Autodesk Inventor part; units mm, degrees
ref_plane "YZ Plane" through (0, 0, 0) normal (1, 0, 0) x (0, 1, 0)
ref_plane "XZ Plane" through (0, 0, 0) normal (0, 1, 0) x (-1, 0, 0)
ref_plane "XY Plane" through (0, 0, 0) normal (0, 0, 1) x (1, 0, 0)
sketch "スケッチ1" plane through (0, 0, 0) normal (0, 1, 0) x (-1, 0, 0)
  line L0 (19, -14) -> (-19, -14)
  line L1 (-19, -14) -> (-19, 14)
  line L2 (-19, 14) -> (19, 14)
  line L3 (19, 14) -> (19, -14)
  line L4 (0, -29.0161) -> (0, 0) construction
  line L5 (0, 0) -> (-35.7009, 0) construction
  dimension "d0" = 28
  dimension "d1" = 38
extrude "押し出し1" add sketch "スケッチ1" along normal blind 9
sketch "スケッチ2" plane through (19, 0, 14) normal (1, 0, 0) x (0, 0, -1)
  circle A0 centre (4, 4.5) radius 3.2
  circle A1 centre (24, 4.5) radius 3.2
  line L0 (14, 0) -> (14, 13.3694) construction
  line L1 (0, 0) -> (28, 0)
  dimension "d4" = 6.4
  dimension "d5" = 6.4
  dimension "d6" = 20
  dimension "d7" = 4.5
extrude "押し出し2" cut sketch "スケッチ2" against normal through all
sketch "スケッチ3" plane through (0, 9, 0) normal (0, 1, 0) x (1, 0, 0)
  circle A0 centre (0, 0) radius 12.5
  dimension "d10" = 25
extrude "押し出し3" cut sketch "スケッチ3" against normal blind 0.3
sketch "スケッチ4" plane through (0, 9, 0) normal (0, 1, 0) x (1, 0, 0)
  circle A0 centre (-16, 0) radius 1.5
  circle A1 centre (16, 0) radius 1.5
  line L0 (-19, 14) -> (-19, -14)
  line L1 (19, -14) -> (19, 14)
  point P0 (0, 0)
  dimension "d13" = 3
  dimension "d14" = 3
  dimension "d15" = 3
  dimension "d16" = 3
extrude "押し出し4" cut sketch "スケッチ4" against normal through all
thread "ねじ1"
thread "ねじ2"
properties part number "HayashiProbeHead_sub" material "ステンレス鋼 440C"
Can you work these out from the model? Positions are in its coordinate system, mm. A direction names the side the tool comes from. Give positions to 0.01 mm unless a question says otherwise; leave off trailing zeros. Order: outer loops, then holes, each group sorted by start corner. A loop starts at its lowest first (then second) coordinate and runs counter-clockwise, first axis right, second up. Notation, with made-up numbers: M -5,35 L 13,35 A14 cw 13,60 Z; hole C 28,81 d1. An arc over 180 degrees is marked long. Use a Markdown table: item, result. Add a question column.
Item 1: If I drill on L1, parallel to X at y = 4, z = 0; L2, parallel to Y at x = -10, z = 10; L3, parallel to Z at x = -15.5, y = 6, over which ranges is the centre line in solid material (lowest first)? Write a range as [from, to].
Item 2: Suppose I cut it at A-A (x = 16). List the corners of the cut face in (y, z) for me, then the cut area to 3 significant figures.
Item 3: We'd pull the mould along Z, two halves only. Please class faces 3 (the cylindrical face through (5.77, 8.85, 11.09)), 4 (the cylindrical face through (0.3, 4.6, 13.2)), 5 (the flat face through (0, 4, -14)), 6 (the flat face through (0, 0, 0)): +Z half, -Z half, draft (parallel to the pull), parting line (faces both ways), or undercut.
Item 4: Suppose I cut it at C-C (y = 5). List the corners of the cut face in (x, z) for me.
Item 5: For faces 1 (the flat face through (-19, 4, 0)), 2 (the flat face through (0, 8.7, 0)), which set-ups out of +Z, -Z, +X, -X, +Y, -Y let a thin tool reach every point of the face, with its end or its side?
Item 6: Will these pins go through, and if not, where does the flat tip stop? pin 1 (12 mm diameter, centred on x = -3, z = -6.5, fed in from +Y); pin 2 (2.5 mm diameter, centred on x = -16, z = 0, fed in from +Y).
Item 7: Suppose I cut it at D-D (z = 0). List the corners of the cut face in (x, y) for me.
Item 8: Suppose I cut it at B-B (z = 10). List the corners of the cut face in (x, y) for me.
Answer sheet:
| question | item | result |
|---|---|---|
| 1 | L1 | x = [-19, -17.5], [-14.5, 14.5], [17.5, 19] |
| 1 | L2 | y = [0, 1.3], [7.7, 9] |
| 1 | L3 | z = [-14, -12.83], [-7.17, -1.41], [1.41, 7.17], [12.83, 14] |
| 2 | outline | M 0,-14 L 9,-14 L 9,-1.5 L 0,-1.5 Z; M 0,1.5 L 9,1.5 L 9,14 L 0,14 Z; hole C 4.5,-10 d6.4; hole C 4.5,10 d6.4 |
| 2 | area | 161 mm² |
| 3 | face 3 | undercut |
| 3 | face 4 | undercut |
| 3 | face 5 | -Z half |
| 3 | face 6 | draft |
| 4 | outline | M -19,-14 L 19,-14 L 19,-13.16 L -19,-13.16 Z; M -19,-6.84 L 19,-6.84 L 19,6.84 L -19,6.84 Z; M -19,13.16 L 19,13.16 L 19,14 L -19,14 Z; hole C -16,0 d3; hole C 16,0 d3 |
| 5 | face 1 | +Z, -Z, -X, +Y, -Y |
| 5 | face 2 | +Y |
| 6 | pin 1 | stops at y = 9 |
| 6 | pin 2 | passes through |
| 7 | outline | M -19,0 L -17.5,0 L -17.5,9 L -19,9 Z; M -14.5,0 L 14.5,0 L 14.5,9 L 12.5,9 L 12.5,8.7 L -12.5,8.7 L -12.5,9 L -14.5,9 Z; M 17.5,0 L 19,0 L 19,9 L 17.5,9 Z |
| 8 | outline | M -19,0 L 19,0 L 19,1.3 L -19,1.3 Z; M -19,7.7 L 19,7.7 L 19,9 L 7.5,9 L 7.5,8.7 L -7.5,8.7 L -7.5,9 L -19,9 Z |
